Here's the drawing with two shaded views (mm, measured from the low corner). I have some questions. A direction names the side the tool comes from. Round coordinates to 2 decimals unless told otherwise and drop trailing zeros. Loops run counter-clockwise (first coordinate to the right, second up) from the corner with the lowest first, then second, coordinate; pieces in that order, holes last. Notation, with made-up numbers: M -30.5,30 L 24.5,30 A26 cw 24.5,48 Z; hole C 25,-5 d11. An arc over 180 degrees is marked long. Write each question's results on one line, items separated by ' | '. Start each with the question number.
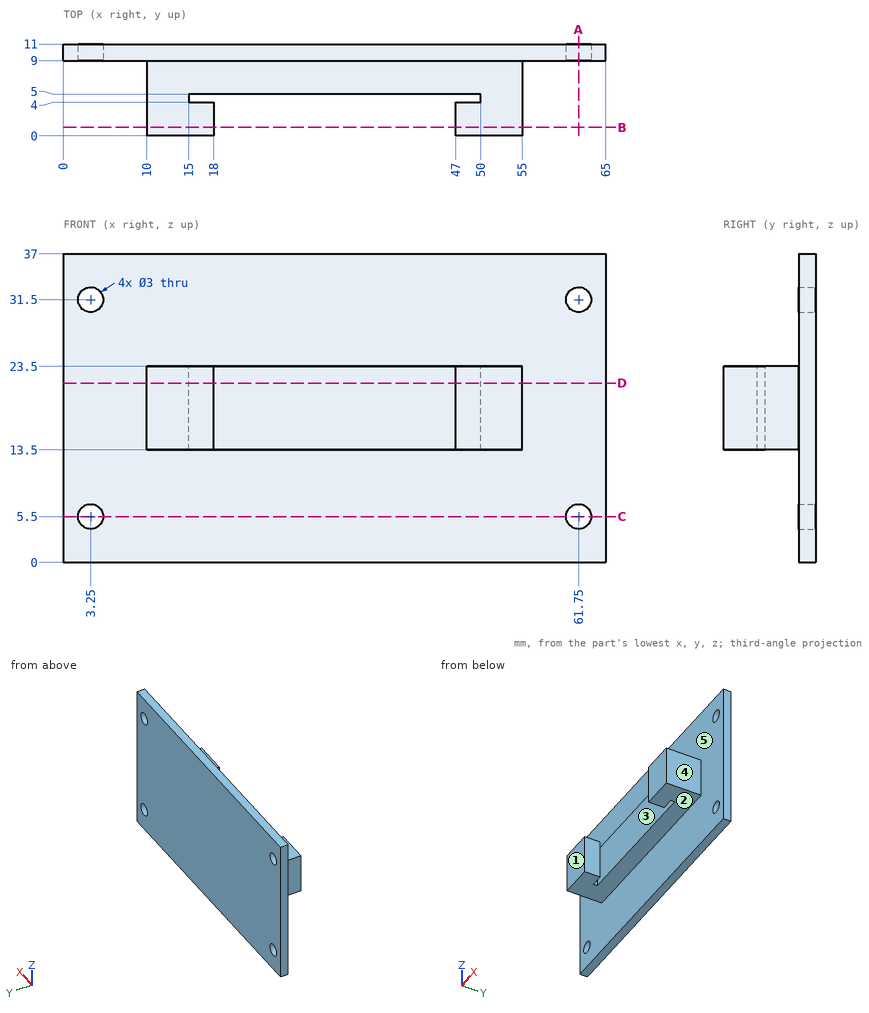
Item 1: If we section it at A-A on x = 61.75: Please give me the cut outline in (y, z).
Item 2: Which directions (+Z, -Z, +X, -X, +Y, -Y) give clear straight access to the entire face, cutting with the end or side of a thin tool? Please do the marked faces 1 and 2.
Item 3: I need wall thicknesses on L1, parallel to X at y = 10.05, z = 5.5; L2, parallel to Z at x = 61.75, y = 10.05; L3, parallel to Y at x = 23, z = 20.5. Which ranges of each line are inside material? Lowest first, please.
Item 4: I'm going to push flat-ended pins straight in: pin 1 (1.2 mm diameter, centred on y = 1.5, z = 20.5, fed in from -X); pin 2 (4.5 mm diameter, centred on x = 31.5, y = 6, fed in from +Z); pin 3 (2.5 mm diameter, centred on x = 3.25, z = 31.5, fed in from -Y); pin 4 (5 mm diameter, centred on x = 61.75, z = 31.5, fed in from -Y). Where does each tip first touch, or does it pass through?
Item 5: If we section it at D-D on z = 21.5: Please give me the cut outline in (x, y), and give its area (3 significant figures).
Item 6: If we section it at C-C on z = 5.5: Please give me the cut outline in (x, y).
Item 7: If we section it at B-B on y = 1: Please give me the cut outline in (x, z), and give its area (3 significant figures).
Item 8: If we mould it in two halves opening along X, with no side actions, what happens to the marked faces 3, 4 and 5? For each: released by +X, released by -X, zero draft, split by the parting line, or undercut.
Numbers:
1) outline: M 9,0 L 11,0 L 11,4 L 9,4 Z; M 9,7 L 11,7 L 11,30 L 9,30 Z; M 9,33 L 11,33 L 11,37 L 9,37 Z
2) face 1: +Z, -Z, +X, -X, -Y | face 2: -Z, +X, -X, -Y
3) L1: 0 to 1.75, 4.75 to 60.25, 63.25 to 65 | L2: 0 to 4, 7 to 30, 33 to 37 | L3: 5 to 11
4) pin 1: x = 10 | pin 2: z = 23.5 | pin 3: through | pin 4: y = 9
5) outline: M 0,9 L 10,9 L 10,0 L 18,0 L 18,4 L 15,4 L 15,5 L 50,5 L 50,4 L 47,4 L 47,0 L 55,0 L 55,9 L 65,9 L 65,11 L 0,11 Z | area: 384 mm²
6) outline: M 0,9 L 1.75,9 L 1.75,11 L 0,11 Z; M 4.75,9 L 60.25,9 L 60.25,11 L 4.75,11 Z; M 63.25,9 L 65,9 L 65,11 L 63.25,11 Z
7) outline: M 10,13.5 L 18,13.5 L 18,23.5 L 10,23.5 Z; M 47,13.5 L 55,13.5 L 55,23.5 L 47,23.5 Z | area: 160 mm²
8) face 3: undercut | face 4: released by +X | face 5: zero draft
